CAD build for the part. Positions are in the model's coordinates, mm. A direction names the side the tool comes from. Coordinates: 2 decimals unless noted, no trailing zeros. Loops run counter-clockwise (first coordinate to the right, second up) from the corner with the lowest first, then second, coordinate; pieces in that order, holes last. Notation, with made-up numbers: (-13, 32) -> (24, 32) arc R22 cw to (24, 38) -> close; hole circle Ø9 at (5, 81). An arc over 180 degrees is marked (long way). Return JSON: item names as keys, results as strings. Group by question number.
(1) Saw through at A-A on z = 13. Write the cut outline in (x, y).
(2) Tool access for faces 1 (the face through (-21.15, 0, 21)), 2 (the face through (-10, -9, 0)): list every direction of +Z, -Z, +X, -X, +Y, -Y with a clear straight run to the whole face (end or side of a thin tool).
(3) Mould opens along Y. For faces 3 (the face through (14, -15.43, 20.71)), 4 (the face through (0, 0, -24)), 5 (the face through (-2.5, -0.1, -12.8)) say: pulls with the +Y half, pulls with the -Y half, needs draft (parallel to the pull), parting line crosses it, or undercut.
(4) Saw through at B-B on x = 0. Write the cut outline in (y, z).
(5) Probe L1, parallel to Y at x = 15.5, z = 39.5; L2, parallel to Y at x = -15, z = 12; L3, parallel to Z at x = 9, y = -4. List the from-to ranges inside material, lowest first.
(6) Flat gauge pin, fed straight in: pin 1 Ø1 at (x, y) = (14, 4.5) entering from -Z. Where does the tip first touch, or does it go through?
(7) Saw through at D-D on z = -11. Write the cut outline in (x, y).
```python
from build123d import *

# Parameters (mm, degrees)
SKETCH1_R           = 1.5
BOSS_EXTRUDE1_DEPTH = 42


with BuildPart() as part:
    # Sketch1 → Boss-Extrude1 (new body)
    with BuildSketch(Plane.XY):
        Polygon((-15.5, 21.15), (-21.15, 15.5), (-21.15, -15.5), (-15.5, -21.15), (15.5, -21.15), (21.15, -15.5), (21.15, 15.5), (15.5, 21.15), align=None)
        with Locations((15.5, 15.5)):
            Circle(SKETCH1_R, mode=Mode.SUBTRACT)
        with Locations((15.5, -15.5)):
            Circle(SKETCH1_R, mode=Mode.SUBTRACT)
        with Locations((-15.5, -15.5)):
            Circle(SKETCH1_R, mode=Mode.SUBTRACT)
        with Locations((-15.5, 15.5)):
            Circle(SKETCH1_R, mode=Mode.SUBTRACT)
    extrude(amount=BOSS_EXTRUDE1_DEPTH)

    # Sketch3 → Revolve1 (revolve)
    with BuildSketch(Plane(origin=(0, 0, 0), x_dir=(0, 0, -1), z_dir=(1, 0, 0)), mode=Mode.PRIVATE) as revolve1_sk:
        Polygon((0, 0), (24, 0), (24, 2.5), (2, 2.5), (2, 11), (0, 11), align=None)
    revolve(revolve1_sk.sketch.rotate(Axis((0, 0, 0), (0, 0, -1)), 90), axis=Axis((0, 0, 0), (0, 0, -1)))


solid = part.part
```
Geometry results:
{
 "1": {"outline": "(-21.15, -15.5) -> (-15.5, -21.15) -> (15.5, -21.15) -> (21.15, -15.5) -> (21.15, 15.5) -> (15.5, 21.15) -> (-15.5, 21.15) -> (-21.15, 15.5) -> close; hole circle Ø3 at (-15.5, -15.5); hole circle Ø3 at (-15.5, 15.5); hole circle Ø3 at (15.5, -15.5); hole circle Ø3 at (15.5, 15.5)"},
 "2": {"face 1": "+Z, -Z, -X, +Y, -Y", "face 2": "-Z"},
 "3": {"face 3": "undercut", "face 4": "needs draft", "face 5": "parting line crosses it"},
 "4": {"outline": "(-21.15, 0) -> (-11, 0) -> (-11, -2) -> (-2.5, -2) -> (-2.5, -24) -> (2.5, -24) -> (2.5, -2) -> (11, -2) -> (11, 0) -> (21.15, 0) -> (21.15, 42) -> (-21.15, 42) -> close"},
 "5": {"L1": "-21.15 to -17, -14 to 14, 17 to 21.15", "L2": "-21.15 to -16.91, -14.09 to 14.09, 16.91 to 21.15", "L3": "-2 to 42"},
 "6": {"pin 1": "z = 0"},
 "7": {"outline": "circle Ø5 at (0, 0)"}
}
